```python
from build123d import *

# Parameters (mm, degrees)
SKETCH2_W           = 63
SKETCH2_H           = 96
BOSS_EXTRUDE1_DEPTH = 5
SKETCH3_R           = 2.1
CUT_EXTRUDE1_DEPTH  = 5
SKETCH4_W           = 28
SKETCH4_H           = 72
BOSS_EXTRUDE2_DEPTH = 5


with BuildPart() as part:
    # Sketch2 → Boss-Extrude1 (new body)
    with BuildSketch(Plane.XY):
        with Locations((31.5, 48)):
            Rectangle(SKETCH2_W, SKETCH2_H)
    extrude(amount=BOSS_EXTRUDE1_DEPTH)

    # Sketch3 → Cut-Extrude1 (cut)
    with BuildSketch(Plane.XY.offset(5)):
        with Locations((14, 91)):
            Circle(SKETCH3_R)
        with Locations(Location((49, 91, 0), (0, 0, 180))):
            Circle(SKETCH3_R)
        with Locations((49, 5)):
            Circle(SKETCH3_R)
        with Locations(Location((14, 5, 0), (0, 0, 180))):
            Circle(SKETCH3_R)
    extrude(amount=-CUT_EXTRUDE1_DEPTH, mode=Mode.SUBTRACT)

    # Sketch4 → Boss-Extrude2 (add)
    with BuildSketch(Plane.XY.offset(5)):
        with Locations((77, 48)):
            Rectangle(SKETCH4_W, SKETCH4_H)
        with Locations((-14, 48)):
            Rectangle(SKETCH4_W, SKETCH4_H)
    extrude(amount=-BOSS_EXTRUDE2_DEPTH)


solid = part.part
```
Could you check a few things on this model? Use its own coordinates, in mm. A direction names the side the tool comes from. Give positions to 0.01 mm unless a question says otherwise; leave off trailing zeros. Order: outer loops, then holes, each group sorted by start corner. A loop starts at its lowest first (then second) coordinate and runs counter-clockwise, first axis right, second up.
Q1. Suppose I cut it at C-C, the plane x = 49. Write out the boundary of the cut face in (y, z), and give its area (3 significant figures).
Q2. I'm going to push flat-ended pins straight in: P1, Ø2.5, axis at x = 71, z = 2.5, coming from the -Y side; P2, Ø2.5, axis at x = -16, z = 3.5, coming from the +Y side. Where does each tip first touch, or does it pass through?
Q3. Suppose I cut it at D-D, the plane y = 9. Write out the boundary of the cut face in (x, z), and give its area (3 significant figures).
Q4. For faces 1 (the flat face through (0, 6, 2)), 2 (the flat face through (-14, 84, 3)), 3 (the flat face through (77, 12, 3)), 4 (the flat face through (63, 90, 2)), 5 (the cylindrical face through (51.003, 5.631, 2.535)), which set-ups out of +Z, -Z, +X, -X, +Y, -Y let a thin tool reach every point of the face, with its end or its side?
Q5. Suppose I cut it at B-B, the plane y = 91. Write out the boundary of the cut face in (x, z), and give its area (3 significant figures).
Q6. Suppose I cut it at A-A, the plane z = 3.2. Write out the boundary of the cut face in (x, y), and give its area (3 significant figures).
Q7. If I drill on line 1 along Y through (x, z) = (49, 1.7); line 2 along Y through (x, z) = (84.5, 0.75); line 3 along X through (y, z) = (8, 1.55), over which ranges is the centre line in solid material (lowest first)?
Q8. We'd pull the mould along Y, two halves only. Please class faces 6 (the cylindrical face through (14.46, 7.05, 2.54)), 7 (the flat face through (-14, 12, 3)), 8 (the flat face through (63, 6, 2)): +Y half, -Y half, draft (parallel to the pull), parting line (faces both ways), or undercut.
Solution:
1. outline: (0, 0) - (2.9, 0) - (2.9, 5) - (0, 5) - close; (7.1, 0) - (88.9, 0) - (88.9, 5) - (7.1, 5) - close; (93.1, 0) - (96, 0) - (96, 5) - (93.1, 5) - close
1. area: 438 mm2
2. P1: stops at y = 12
2. P2: stops at y = 84
3. outline: (0, 0) - (63, 0) - (63, 5) - (0, 5) - close
3. area: 315 mm2
4. face 1: +Z, -Z, -X, -Y
4. face 2: +Z, -Z, -X, +Y
4. face 3: +Z, -Z, +X, -Y
4. face 4: +Z, -Z, +X, +Y
4. face 5: +Z, -Z
5. outline: (0, 0) - (11.9, 0) - (11.9, 5) - (0, 5) - close; (16.1, 0) - (46.9, 0) - (46.9, 5) - (16.1, 5) - close; (51.1, 0) - (63, 0) - (63, 5) - (51.1, 5) - close
5. area: 273 mm2
6. outline: (-28, 12) - (0, 12) - (0, 0) - (63, 0) - (63, 12) - (91, 12) - (91, 84) - (63, 84) - (63, 96) - (0, 96) - (0, 84) - (-28, 84) - close; hole circle Ø4.2 at (14, 5); hole circle Ø4.2 at (14, 91); hole circle Ø4.2 at (49, 5); hole circle Ø4.2 at (49, 91)
6. area: 10,000 mm2
7. line 1: y = 0 to 2.9, 7.1 to 88.9, 93.1 to 96
7. line 2: y = 12 to 84
7. line 3: x = 0 to 63
8. face 6: undercut
8. face 7: -Y half
8. face 8: draft
